```python
from build123d import *

# Parameters (mm, degrees)
F0_W     = 152.4
F0_H     = 1524
F0_W_2   = 114.3
F0_H_2   = 1485.9
F1_DEPTH = 1828.8
F3_DEPTH = 25.4
F5_DEPTH = 25.4


with BuildPart() as f1:
    # F0 (on Top) → F1 (new body)
    with BuildSketch(Plane.XY):
        Rectangle(F0_W, F0_H)
        Rectangle(F0_W_2, F0_H_2, mode=Mode.SUBTRACT)
    extrude(amount=F1_DEPTH)

    # F2 (on face) → F3 (cut)
    with BuildSketch(Plane.YZ.offset(76.2)):
        Polygon((-133.35, 101.6), (0, 101.6), (0, 260.35), (0, 419.1), (-133.35, 419.1), align=None)
        Polygon((0, 260.35), (0, 101.6), (133.35, 101.6), (133.35, 419.1), (0, 419.1), align=None)
        with BuildLine():
            ThreePointArc((30.1625, 660.4), (-21.328108, 681.728108), (0, 630.2375))
            ThreePointArc((0, 630.2375), (21.328108, 639.071892), (30.1625, 660.4))
        make_face()
        with BuildLine():
            ThreePointArc((30.1625, 1320.8), (21.328108, 1342.128108), (0, 1350.9625))
            ThreePointArc((0, 1350.9625), (-21.328108, 1299.471892), (30.1625, 1320.8))
        make_face()
    extrude(amount=-F3_DEPTH, mode=Mode.SUBTRACT)

    # F4 (on face) → F5 (cut)
    with BuildSketch(Plane(origin=(-76.2, 0, 0), x_dir=(0, -1, 0), z_dir=(-1, 0, 0))):
        with BuildLine():
            ThreePointArc((30.1625, 1320.8), (21.328108, 1342.128108), (0, 1350.9625))
            ThreePointArc((0, 1350.9625), (-21.328108, 1299.471892), (30.1625, 1320.8))
        make_face()
        with BuildLine():
            ThreePointArc((30.1625, 660.4), (-21.328108, 681.728108), (0, 630.2375))
            ThreePointArc((0, 630.2375), (21.328108, 639.071892), (30.1625, 660.4))
        make_face()
    extrude(amount=-F5_DEPTH, mode=Mode.SUBTRACT)


solid = f1.part
```
CAD build for the part. Positions are in the model's coordinates, mm. A direction names the side the tool comes from. Round coordinates to 2 decimals unless told otherwise and drop trailing zeros. Order: outer loops, then holes, each group sorted by start corner. A loop starts at its lowest first (then second) coordinate and runs counter-clockwise, first axis right, second up.
Item 1: Saw through at C-C on z = 1394. Write the cut outline in (x, y).
Item 2: Probe line 1 along Z through (x, y) = (66, 0); line 2 along Y through (x, z) = (-56.5, 1156); line 3 along X through (y, z) = (196, 876.5). List the from-to ranges inside material, lowest first.
Item 3: Mould opens along X. For faces 3 (the face through (62, 4, 0)), 4 (the face through (-1, 742.95, 902)), 5 (the face through (-76.2, -11, 902)) say: pulls with the +X half, pulls with the -X half, needs draft (parallel to the pull), parting line crosses it, or undercut.
Item 4: Saw through at B-B on y = -528. Write the cut outline in (x, z), then the cut area to 3 significant figures.
Item 5: Tool access for faces 1 (the face through (-1, -762, 902)), 2 (the face through (57.15, -10, 902)): list every direction of +Z, -Z, +X, -X, +Y, -Y with a clear straight run to the whole face (end or side of a thin tool).
Item 6: Saw through at D-D on z = 261. Write the cut outline in (x, y).
Item 7: Saw through at A-A on x = 5.5. Write the cut outline in (y, z), then the cut area to 3 significant figures.
Reported:
1. outline: (-76.2, -762) - (76.2, -762) - (76.2, 762) - (-76.2, 762) - close; hole (-57.15, -742.95) - (57.15, -742.95) - (57.15, 742.95) - (-57.15, 742.95) - close
2. line 1: z = 0 to 101.6, 419.1 to 630.24, 690.56 to 1290.64, 1350.96 to 1828.8
2. line 2: y = -762 to -742.95, 742.95 to 762
2. line 3: x = -76.2 to -57.15, 57.15 to 76.2
3. face 3: needs draft
3. face 4: undercut
3. face 5: pulls with the -X half
4. outline: (-76.2, 0) - (-57.15, 0) - (-57.15, 1828.8) - (-76.2, 1828.8) - close; (57.15, 0) - (76.2, 0) - (76.2, 1828.8) - (57.15, 1828.8) - close
4. area: 69,700 mm2
5. face 1: +Z, -Z, +X, -X, -Y
5. face 2: +Z, -Z
6. outline: (-76.2, -762) - (76.2, -762) - (76.2, -133.35) - (57.15, -133.35) - (57.15, -742.95) - (-57.15, -742.95) - (-57.15, 742.95) - (57.15, 742.95) - (57.15, 133.35) - (76.2, 133.35) - (76.2, 762) - (-76.2, 762) - close
7. outline: (-762, 0) - (-742.95, 0) - (-742.95, 1828.8) - (-762, 1828.8) - close; (742.95, 0) - (762, 0) - (762, 1828.8) - (742.95, 1828.8) - close
7. area: 69,700 mm2
